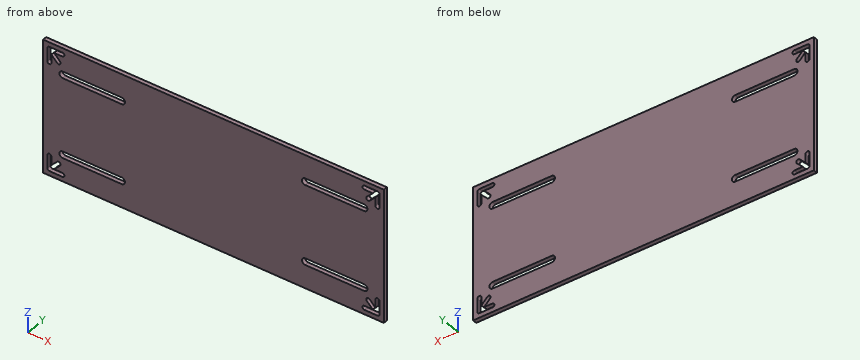
```python
from build123d import *

# Parameters (mm, degrees)
SKETCH1_W            = 260
SKETCH1_H            = 100
BASE_DEPTH           = 3.175
SLOTS_DEPTH          = 140.320065407
MOUNT_HOLES_DEPTH    = 3.175
MIRROR2_COPY_1_DEPTH = 3.175


with BuildPart() as part:
    # Sketch1 → Base (new body)
    with BuildSketch(Plane(origin=(0, 0, 0), x_dir=(1, 0, 0), z_dir=(0, 1, 0))):
        Rectangle(SKETCH1_W, SKETCH1_H)
    extrude(amount=BASE_DEPTH)

    # Sketch2 → Slots (cut, through all)
    with BuildSketch(Plane(origin=(0, 3.175, 0), x_dir=(1, 0, 0), z_dir=(0, 1, 0))):
        with BuildLine():
            Line((-115, 32.5), (-70, 32.5))
            ThreePointArc((-70, 32.5), (-67.5, 30), (-70, 27.5))
            Line((-70, 27.5), (-115, 27.5))
            ThreePointArc((-115, 27.5), (-117.5, 30), (-115, 32.5))
        make_face()
        with BuildLine():
            Line((-115, -32.5), (-70, -32.5))
            ThreePointArc((-70, -32.5), (-67.5, -30), (-70, -27.5))
            Line((-70, -27.5), (-115, -27.5))
            ThreePointArc((-115, -27.5), (-117.5, -30), (-115, -32.5))
        make_face()
        with BuildLine():
            Line((115, 32.5), (70, 32.5))
            ThreePointArc((70, 32.5), (67.5, 30), (70, 27.5))
            Line((70, 27.5), (115, 27.5))
            ThreePointArc((115, 27.5), (117.5, 30), (115, 32.5))
        make_face()
        with BuildLine():
            Line((115, -32.5), (70, -32.5))
            ThreePointArc((70, -32.5), (67.5, -30), (70, -27.5))
            Line((70, -27.5), (115, -27.5))
            ThreePointArc((115, -27.5), (117.5, -30), (115, -32.5))
        make_face()
    extrude(amount=-SLOTS_DEPTH, mode=Mode.SUBTRACT)

    # Sketch3 → Mount Holes (cut)
    with BuildSketch(Plane(origin=(0, 3.175, 0), x_dir=(1, 0, 0), z_dir=(0, 1, 0))):
        with BuildLine():
            Line((-125.150208204, 46.650208204), (-115.150208204, 46.650208204))
            ThreePointArc((-115.150208204, 46.650208204), (-113.650208204, 45.150208204), (-115.150208204, 43.650208204))
            Line((-115.150208204, 43.650208204), (-121.528887861, 43.650208204))
            Line((-121.528887861, 43.650208204), (-117.018480221, 39.139800564))
            ThreePointArc((-117.018480221, 39.139800564), (-117.018480221, 37.018480221), (-119.139800564, 37.018480221))
            Line((-119.139800564, 37.018480221), (-123.650208204, 41.528887861))
            Line((-123.650208204, 41.528887861), (-123.650208204, 35.150208204))
            ThreePointArc((-123.650208204, 35.150208204), (-125.150208204, 33.650208204), (-126.650208204, 35.150208204))
            Line((-126.650208204, 35.150208204), (-126.650208204, 45.150208204))
            ThreePointArc((-126.650208204, 45.150208204), (-126.210868376, 46.210868376), (-125.150208204, 46.650208204))
        make_face()
    mount_holes = extrude(amount=-MOUNT_HOLES_DEPTH, mode=Mode.SUBTRACT)

    # Mirror1: Mount Holes across plane
    add(mount_holes.mirror(Plane(origin=(0, 0, 0), x_dir=(0, 0, 1), z_dir=(1, 0, 0))), mode=Mode.SUBTRACT)

    # Mirror2: Mount Holes across plane
    add(mount_holes.mirror(Plane.XY), mode=Mode.SUBTRACT)

    # Mirror2 copy 1 sketch → Mirror2 copy 1 (cut)
    with BuildSketch(Plane(origin=(0, 3.175, 0), x_dir=(-1, 0, 0), z_dir=(0, 1, 0))):
        with BuildLine():
            Line((-125.150208204, 46.650208204), (-115.150208204, 46.650208204))
            ThreePointArc((-115.150208204, 46.650208204), (-113.650208204, 45.150208204), (-115.150208204, 43.650208204))
            Line((-115.150208204, 43.650208204), (-121.528887861, 43.650208204))
            Line((-121.528887861, 43.650208204), (-117.018480221, 39.139800564))
            ThreePointArc((-117.018480221, 39.139800564), (-117.018480221, 37.018480221), (-119.139800564, 37.018480221))
            Line((-119.139800564, 37.018480221), (-123.650208204, 41.528887861))
            Line((-123.650208204, 41.528887861), (-123.650208204, 35.150208204))
            ThreePointArc((-123.650208204, 35.150208204), (-125.150208204, 33.650208204), (-126.650208204, 35.150208204))
            Line((-126.650208204, 35.150208204), (-126.650208204, 45.150208204))
            ThreePointArc((-126.650208204, 45.150208204), (-126.210868376, 46.210868376), (-125.150208204, 46.650208204))
        make_face()
    extrude(amount=-MIRROR2_COPY_1_DEPTH, mode=Mode.SUBTRACT)


solid = part.part
```
Build history of the part. All positions in model axes, mm. Round coordinates to 2 decimals unless told otherwise and drop trailing zeros. Loops run counter-clockwise (first coordinate to the right, second up) from the corner with the lowest first, then second, coordinate; pieces in that order, holes last.
Item 1: Drill centre lines: line 1 along Z through (x, y) = (-90, 1.3); line 2 along X through (y, z) = (2.15, 35); line 3 along X through (y, z) = (0.9, -34.5). Where is each one in solid material? Low to high.
Item 2: Saw through at C-C (y = 1.25). State how many separate pieces and enclosed holes the cut face has, then the cut area to 3 significant figures.
Item 3: Saw through at A-A (z = -30). List the corners of the cut face in (x, y) (3 decimals), then the cut area to 3 significant figures.
Item 4: Saw through at B-B (x = -98). List the corners of the cut face in (y, z) (3 decimals), then the cut area to 3 significant figures.
Worked answers:
1. line 1: z = -50 to -32.5, -27.5 to 27.5, 32.5 to 50
1. line 2: x = -130 to -126.64, -123.66 to 123.66, 126.64 to 130
1. line 3: x = -130 to -126.5, -123.8 to 123.8, 126.5 to 130
2. separate pieces: 1
2. enclosed holes: 8
2. area: 24,700 mm2
3. outline: (-130, 0) - (-117.5, 0) - (-117.5, 3.175) - (-130, 3.175) - close; (-67.5, 0) - (67.5, 0) - (67.5, 3.175) - (-67.5, 3.175) - close; (117.5, 0) - (130, 0) - (130, 3.175) - (117.5, 3.175) - close
3. area: 508 mm2
4. outline: (0, -50) - (3.175, -50) - (3.175, -32.5) - (0, -32.5) - close; (0, -27.5) - (3.175, -27.5) - (3.175, 27.5) - (0, 27.5) - close; (0, 32.5) - (3.175, 32.5) - (3.175, 50) - (0, 50) - close
4. area: 286 mm2
